Autodesk Inventor part; units mm, degrees
ref_plane "YZ Plane" through (0, 0, 0) normal (1, 0, 0) x (0, 1, 0)
ref_plane "XZ Plane" through (0, 0, 0) normal (0, 1, 0) x (-1, 0, 0)
ref_plane "XY Plane" through (0, 0, 0) normal (0, 0, 1) x (1, 0, 0)
sketch "Sketch1" plane through (0, 0, 0) normal (0, 0, 1) x (1, 0, 0)
  line L0 (0, 0) -> (-20, 0)
  line L1 (-20, 0) -> (-20, 3.4)
  line L2 (-20, 3.4) -> (-16, 3.4)
  line L3 (-16, 3.4) -> (-16, 2)
  line L4 (-16, 2) -> (0, 2)
  line L5 (0, 2) -> (0, 0)
  dimension "d0" = 4
  dimension "d1" = 2
  dimension "d2" = 20
  dimension "d3" = 3.4
revolve "Revolution1" add sketch "Sketch1" angle 360 about axis through (0, 0, 0) along (-1, 0, 0)
fillet "Fillet1" radius 0.3 1 edges at (-20, -3.4, 0)
chamfer "Chamfer1" distance 0.1 angle 45 1 edges at (-16, -3.4, 0)
thread "Thread1"
sketch "Sketch2" plane through (-20, 0, 0) normal (-1, 0, 0) x (0, 0, 1)
  line L0 (-1.1237, 1.3558) -> (0.6123, 1.651)
  line L1 (0.6123, 1.651) -> (1.736, 0.2952)
  line L2 (1.736, 0.2952) -> (1.1237, -1.3558)
  line L3 (1.1237, -1.3558) -> (-0.6123, -1.651)
  line L4 (-0.6123, -1.651) -> (-1.736, -0.2952)
  line L5 (-1.736, -0.2952) -> (-1.1237, 1.3558)
  point P0 (0, 0)
  point P1 (0, 0)
  dimension "d11" = 3.05
extrude "Extrusion1" cut sketch "Sketch2" against normal blind 2.5
properties part number "Screw_StainlessSteal_M4_SocketCap_20mm" material "Stainless Steel"
Part model, mm, in its own coordinate system. A direction names the side the tool comes from. Coordinates: 2 decimals unless noted, no trailing zeros. Loops run counter-clockwise (first coordinate to the right, second up) from the corner with the lowest first, then second, coordinate; pieces in that order, holes last. Notation, with made-up numbers: M 22,41.25 L 76,41.25 A30 ccw 76,74.25 Z; hole C 16,66 d5. An arc over 180 degrees is marked long. Use a Markdown table: item, result. Add a question column.
Q1. Probe L1, parallel to X at y = -0.5, z = -2.25; L2, parallel to Y at x = -17, z = 2.75; L3, parallel to Z at x = -14, y = -1. List the from-to ranges inside material, lowest first.
Q2. Cut at A-A (x = -19). Write the cut outline in (y, z).
Q3. Cut at C-C (x = -7.5). Write the cut outline in (y, z).
Q4. Cut at B-B (y = 0). Write the cut outline in (x, z), and give its area (3 significant figures).
Q5. Mould opens along Y. For faces 4 (the flat face through (-16, 0, 2.2)), 5 (the flat face through (-17.5, 0, 0)), 6 (the cylindrical face through (-17.87, -0.74, -3.32)), 7 (the flat face through (-18.77, 0.98, 1.17)) say: +Y half, -Y half, draft (parallel to the pull), parting line (faces both ways), or undercut.
Q6. Which spindle directions (+Z, -Z, +X, -X, +Y, -Y) get a long thin tool onto all of the face, cutting with end or side? Do faces 1 (the cylindrical face through (-8, 0, -2)), 2 (the flat face through (-18.77, -1.5, 0.27)), 3 (the flat face through (0, 0, 0)). Say none if no direction does.
Q7. Pin check, flat tips, straight feed: P1, Ø1, axis at x = -9, y = 1.5, coming from the +Z side; P2, Ø2.5, axis at y = 0.5, z = 0.5, coming from the -X side; P3, Ø1.5, axis at x = -3, z = -1, coming from the +Y side; P4, Ø4, axis at x = -6.5, y = -1, coming from the +Z side. Stop position of each tip, or through.
Worked out:
| question | item | result |
|---|---|---|
| 1 | L1 | x = -20 to -16 |
| 1 | L2 | y = -2 to 2 |
| 1 | L3 | z = -1.73 to 1.73 |
| 2 | outline | C 0,0 d6.8; hole M -1.65,-0.61 L -0.3,-1.74 L 1.36,-1.12 L 1.65,0.61 L 0.3,1.74 L -1.36,1.12 Z |
| 3 | outline | C 0,0 d4 |
| 4 | outline | M -20,-3.1 A0.3 ccw -19.7,-3.4 L -16.1,-3.4 L -16,-3.3 L -16,-2 L 0,-2 L 0,2 L -16,2 L -16,3.3 L -16.1,3.4 L -19.7,3.4 A0.3 ccw -20,3.1 L -20,1.63 L -17.5,1.63 L -17.5,-1.63 L -20,-1.63 Z |
| 4 | area | 83.0 mm2 |
| 5 | face 4 | draft |
| 5 | face 5 | undercut |
| 5 | face 6 | parting line |
| 5 | face 7 | undercut |
| 6 | face 1 | +X |
| 6 | face 2 | -X |
| 6 | face 3 | +Z, -Z, +X, +Y, -Y |
| 7 | P1 | stops at z = 1.73 |
| 7 | P2 | stops at x = -20 |
| 7 | P3 | stops at y = 1.98 |
| 7 | P4 | stops at z = 2 |
